```python
from build123d import *

# Parameters (mm, degrees)
SKETCH1_W                    = 300
SKETCH1_H                    = 178
BOSS_EXTRUDE1_DEPTH          = 3
M5_CLEARANCE_HOLE1_OUTLINE_R = 2.75
M5_CLEARANCE_HOLE1_DEPTH     = 3
SKETCH4_W                    = 25
SKETCH4_H                    = 20
CUT_EXTRUDE1_DEPTH           = 10
FILLET1_R                    = 1.5


# Read off the part's stored shape, not the designer's step: M5 Clearance Hole1
with BuildPart() as part:
    # Sketch1 → Boss-Extrude1 (new body)
    with BuildSketch(Plane.XY):
        with Locations((150, 89)):
            Rectangle(SKETCH1_W, SKETCH1_H)
    extrude(amount=BOSS_EXTRUDE1_DEPTH)

    # M5 Clearance Hole1 outline → M5 Clearance Hole1 (cut)
    with BuildSketch(Plane.XY):
        with Locations((295, 118.385)):
            Circle(M5_CLEARANCE_HOLE1_OUTLINE_R)
        with Locations((5, 118.385)):
            Circle(M5_CLEARANCE_HOLE1_OUTLINE_R)
        with Locations((295, 173)):
            Circle(M5_CLEARANCE_HOLE1_OUTLINE_R)
        with Locations((295, 63.77)):
            Circle(M5_CLEARANCE_HOLE1_OUTLINE_R)
        with Locations((5, 63.77)):
            Circle(M5_CLEARANCE_HOLE1_OUTLINE_R)
        with Locations((5, 173)):
            Circle(M5_CLEARANCE_HOLE1_OUTLINE_R)
        with Locations((85, 173)):
            Circle(M5_CLEARANCE_HOLE1_OUTLINE_R)
        with Locations((215, 173)):
            Circle(M5_CLEARANCE_HOLE1_OUTLINE_R)
    extrude(amount=M5_CLEARANCE_HOLE1_DEPTH, mode=Mode.SUBTRACT)

    # Sketch4 → Cut-Extrude1 (cut)
    with BuildSketch(Plane.XY.offset(3)):
        with Locations((262.5, 158)):
            Rectangle(SKETCH4_W, SKETCH4_H)
    extrude(amount=-CUT_EXTRUDE1_DEPTH, mode=Mode.SUBTRACT)

    # Fillet1
    fillet1_edges = [part.edges().sort_by_distance(p)[0] for p in [
        (250, 148, 1.5),
        (250, 168, 1.5),
        (275, 168, 1.5),
        (275, 148, 1.5),
    ]]
    fillet(fillet1_edges, radius=FILLET1_R)


solid = part.part
```
Part model, mm, in its own coordinate system. Round coordinates to 2 decimals unless told otherwise and drop trailing zeros. Use a Markdown table: item, result.
1) Pull direction X, two halves, no side cores. Call faces 1 (the cylindrical face through (297.62, 64.6, 1.48)), 2 (the flat face through (148, 90, 0)), 3 (the cylindrical face through (217.54, 171.95, 1.48)): pulls with the +X half, pulls with the -X half, needs draft (parallel to the pull), parting line crosses it, or undercut.
The answers:
| item | result |
|---|---|
| face 1 | undercut |
| face 2 | needs draft |
| face 3 | undercut |
2) Probe line 1 (X direction, y = 173, z = 1.4); line 2 (Y direction, x = 5, z = 2.25) (3 decimals); line 3 (Y direction, x = 215, z = 1.35). List the from-to ranges inside material, lowest first. Write a range as [from, to].
The answers:
| item | result |
|---|---|
| line 1 | x = [0, 2.25], [7.75, 82.25], [87.75, 212.25], [217.75, 292.25], [297.75, 300] |
| line 2 | y = [0, 61.02], [66.52, 115.635], [121.135, 170.25], [175.75, 178] |
| line 3 | y = [0, 170.25], [175.75, 178] |
3) Drop flat-ended pins along their axis: pin 1 Ø9 at (x, y) = (215, 173) entering from -Z; pin 2 Ø4.5 at (x, y) = (5, 173) entering from +Z. Give the stop position or say it passes through.
The answers:
| item | result |
|---|---|
| pin 1 | stops at z = 0 |
| pin 2 | passes through |
